Autodesk Inventor part; units mm, degrees
ref_plane "Arbeitsebene1" through (0, 21, 0) normal (0, 1, 0) x (-1, 0, 0)
ref_plane "YZ Plane" through (0, 0, 0) normal (1, 0, 0) x (0, 1, 0)
ref_plane "XY Plane" through (0, 0, 0) normal (0, 0, 1) x (1, 0, 0)
sketch "Skizze1" plane through (0, 0, 0) normal (0, 0, 1) x (1, 0, 0)
  line L0 (-29.4, 0) -> (29.4, 0)
  line L1 (0, -29.4) -> (0, 29.4)
  circle A0 centre (0, 0) radius 21
  dimension "d0" = 42
extrude "Extrusion1" add sketch "Skizze1" along normal blind 25
sketch "Skizze2" plane through (0, 0, 25) normal (0, 0, 1) x (1, 0, 0)
  circle A0 centre (0, 0) radius 21
  circle A1 centre (0, 0) radius 19.5
  dimension "d3" = 39
extrude "Extrusion2" cut sketch "Skizze2" against normal blind 20 contours A1
sketch "Skizze3" plane through (0, 0, 0) normal (0, 0, -1) x (-1, 0, 0)
  circle A0 centre (0, 0) radius 21
  circle A1 centre (0, 0) radius 15
  dimension "d6" = 30
extrude "Extrusion3" cut sketch "Skizze3" against normal through all contours A1
ref_plane "Arbeitsebene1" through (0, 21, 0) normal (0, 1, 0) x (-1, 0, 0)
sketch "Skizze5" plane through (0, 21, 0) normal (0, 1, 0) x (-1, 0, 0)
  line L0 (0, -5) -> (0, 30)
  line L1 (29.4, 0) -> (-29.4, 0)
  line L2 (21, 25) -> (-21, 25)
  point P0 (0, 0)
  point P1 (0, 23)
  dimension "d13" = 2
hole "Bohrung1" at (0, 21, 23) direction (0, -1, 0) diameter 2.4 end through all
pattern_circular "Runde Anordnung1" count 4 over 360 about axis through (0, 0, 0) along (0, 0, 1) of "Bohrung1"
chamfer "Fase1" distance 1 angle 45 1 edges at (15, 0, 5)
sketch "Skizze6" plane through (0, 21, 0) normal (0, 1, 0) x (-1, 0, 0)
  line L0 (29.4, 0) -> (-29.4, 0)
  line L1 (0, -5) -> (0, 30)
  line L2 (-2, 0) -> (2, 0)
  line L3 (2, 0) -> (2, 2)
  line L4 (0, 4) -> (0, 4)
  line L5 (-2, 2) -> (-2, 0)
  arc A0 (2, 2) -> (0, 4) centre (0, 2) ccw
  arc A1 (0, 4) -> (-2, 2) centre (0, 2) ccw
  point P0 (0, 0)
  dimension "d27" = 4
  dimension "d28" = 4
  dimension "d29" = 2
extrude "Extrusion6" cut sketch "Skizze6" against normal through all
pattern_circular "Runde Anordnung2" count 4 over 360 about axis through (0, 0, 0) along (0, 0, 1) of "Extrusion6"
properties part number "13_1087_029"
Geometry check sheet. Reference: the model listing, model coordinates, mm. A direction names the side the tool comes from. Round coordinates to 2 decimals unless told otherwise and drop trailing zeros. Write each loop counter-clockwise with the first axis right and the second up, starting at its lowest first coordinate (ties: lowest second). Pieces come first, ordered by that corner, then holes. Notation, with made-up numbers: (54.5, 41.25) -> (111.5, 41.25) arc R12 cw to (111.5, 58.25) -> close; hole circle Ø10 at (22, -14). An arc over 180 degrees is marked (long way). One line per item, written item: value. Start each with the question number.
(1) Go/stop test with flat-tipped pins: pin 1 Ø2 at (y, z) = (17.5, 0.5) entering from +X; pin 2 Ø1.6 at (x, z) = (17, 1) entering from -Y; pin 3 Ø1.5 at (x, z) = (11, 21) entering from +Y; pin 4 Ø1.4 at (y, z) = (0, 23) entering from -X. Record where each tip stops, or that it passes through.
(2) Cross-section at A-A, the plane z = 23. Record the cut outline in (x, y).
(3) Access from +Z, -Z, +X, -X, +Y, -Y to the whole of each face (thin tool, end or side, straight path). Record for faces 1 (the cylindrical face through (-10.49, -10.72, 1.97)), 2 (the flat face through (-2, -18, 1)), 3 (the cylindrical face through (-2.539, 19.334, 15.14)), 4 (the flat face through (-18, -2, 1)).
(4) Scan lines: line 1 (Z direction, x = 20, y = 0); line 2 (Y direction, x = -10.5, z = 1.5); line 3 (X direction, y = -3, z = 6.5). Record each from-to range of solid material in increasing order. Write a range as [from, to].
(5) Cross-section at B-B, the plane z = 16.75. Record the cut outline in (x, y).
(6) Draft check along X on faces 5 (the flat face through (2, -18, 1)), 6 (the flat face through (2, 18, 1)), 7 (the cylindrical face through (-18, 0, 4)). Enter one of: +X half, -X half, draft (parallel to the pull), parting line (faces both ways), or undercut.
Answer:
1. pin 1: x = 12.99
1. pin 2: y = -13.36
1. pin 3: y = 18.33
1. pin 4: through
2. outline: (-20.97, -1.2) arc R21 ccw to (-1.2, -20.97) -> (-1.2, -19.46) arc R19.5 cw to (-19.46, -1.2) -> close; (-20.97, 1.2) -> (-19.46, 1.2) arc R19.5 cw to (-1.2, 19.46) -> (-1.2, 20.97) arc R21 ccw to start; (1.2, -20.97) arc R21 ccw to (20.97, -1.2) -> (19.46, -1.2) arc R19.5 cw to (1.2, -19.46) -> close; (1.2, 19.46) arc R19.5 cw to (19.46, 1.2) -> (20.97, 1.2) arc R21 ccw to (1.2, 20.97) -> close
3. face 1: +Z, -Z
3. face 2: -Z, +Y, -Y
3. face 3: +Z
3. face 4: -Z, +X, -X
4. line 1: [4, 21.8], [24.2, 25]
4. line 2: [-18.19, -10.71], [10.71, 18.19]
4. line 3: [-20.78, -19.27], [19.27, 20.78]
5. outline: circle Ø42 at (0, 0); hole circle Ø39 at (0, 0)
6. face 5: undercut
6. face 6: undercut
6. face 7: draft
